For this review, take the finished solid that the model builds, in its own axes (mm). Face numbers are marked on the shaded views. Round coordinates to 2 decimals unless told otherwise and drop trailing zeros. Order: outer loops, then holes, each group sorted by start corner. A loop starts at its lowest first (then second) coordinate and runs counter-clockwise, first axis right, second up. Notation, with made-up numbers: M -1.75,-13.75 L 45.25,-13.75 A31 cw 45.25,24.25 Z; hole C 74,-5.5 d3. An arc over 180 degrees is marked long. Use a Markdown table: item, result.
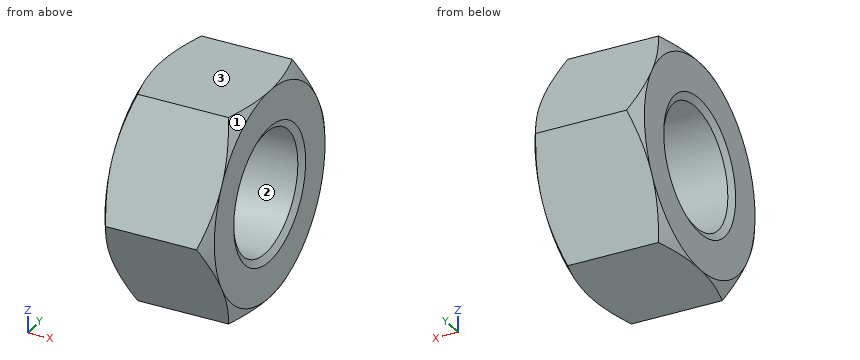
Autodesk Inventor part; units mm, degrees
ref_plane "Work Plane1" through (-87.2182, 0, 0) normal (0, -0.8660254, -0.5) x (1, 0, 0)
ref_plane "YZ Plane" through (0, 0, 0) normal (1, 0, 0) x (0, 1, 0)
ref_plane "XZ Plane" through (0, 0, 0) normal (0, 1, 0) x (-1, 0, 0)
sketch "Sketch1" plane through (0, 0, 0) normal (1, 0, 0) x (0, 1, 0)
  line L0 (-46.188, 0) -> (-23.094, 40)
  line L1 (-23.094, 40) -> (23.094, 40)
  line L2 (23.094, 40) -> (46.188, 0)
  line L3 (46.188, 0) -> (23.094, -40)
  line L4 (23.094, -40) -> (-23.094, -40)
  line L5 (-23.094, -40) -> (-46.188, 0)
  point P0 (0, 0)
  point P1 (0, 0)
  dimension "d0" = 92.376
extrude "Body" add sketch "Sketch1" along normal blind 42
sketch "Sketch2" plane through (0, 0, 0) normal (0, 0, 1) x (1, 0, 0)
  line L0 (0, 23.094) -> (0, 46.188)
  line L1 (0, 46.188) -> (42, 46.188)
  line L2 (42, 23.094) -> (42, 46.188)
  line L3 (-8.4, 0) -> (50.4, 0)
  line L4 (3.5727, 46.188) -> (0, 40)
  line L5 (38.4273, 46.188) -> (42, 40)
  dimension "d3" = 30
  dimension "d4" = 30
  dimension "d5" = 80
  dimension "d6" = 80
revolve "Chamfer1" cut sketch "Sketch2" angle 360 about axis through (-10, 0, 0) along (1, 0, 0)
sketch "Sketch3" plane through (42, 0, 0) normal (1, 0, 0) x (0, 0, -1)
  arc A0 (-20, -34.641) -> (20, -34.641) centre (0, 0) ccw
hole "Thread" at (42, 0, 0) direction (-1, 0, 0) diameter 46.5873 end through all
chamfer "Chamfer2" distance 2.7063 angle 30 1 edges at (42, 0, 23.2937) measured on face at (42, -34.2285, -0.9359)
chamfer "Chamfer3" distance 2.7063 angle 30 1 edges at (0, 0, 23.2937) measured on face at (0, -34.2285, -0.9359)
ref_plane "Work Plane1" through (-87.2182, 0, 0) normal (0, -0.8660254, -0.5) x (1, 0, 0)
equation "\"d0\" = 1.1547 * SW"
equation "\"d1\" = KOH"
equation "\"d8\" = -0.5 * GD1 + 0.5 * NND"
equation "\"d40\" = -0.5 * GD1 + 0.5 * NND"
equation "\"d10\" = -0.5 * GD1 + 0.5 * NND"
equation "\"d41\" = -0.5 * GD1 + 0.5 * NND"
equation "\"d3\" = ANG1"
equation "\"d4\" = ANG2"
equation "\"d5\" = SW0"
equation "\"d6\" = SW01"
equation "\"ANG1\" = 30deg"
equation "\"ANG2\" = ANG1"
equation "\"NND\" = 52"
equation "\"KOH\" = 42"
equation "\"SW0\" = SW"
equation "\"SW01\" = SW"
equation "\"GUL\" = 0.541266 * PTC"
equation "\"THREADDIA\" = 52"
equation "\"TOA\" = 30deg"
equation "\"PTC\" = 5"
equation "\"E0\" = 1.155 * SW"
equation "\"GAL\" = 0.541266 * PTC"
properties part number "BS 3692 - M52" material "Steel, Mild"
Q1. Draft analysis for pull direction Y (two halves, no side actions). For the marked faces 1, 2 and 3, state which applies: pulls with the +Y half, pulls with the -Y half, needs draft (parallel to the pull), parting line crosses it, or undercut.
Determined:
| item | result |
|---|---|
| face 1 | pulls with the -Y half |
| face 2 | undercut |
| face 3 | needs draft |
Q2. Clearance check with flat-ended pins moving along their axes: pin 1 (1.5 mm diameter, centred on x = 7, y = 29, fed in from -Z); pin 2 (4 mm diameter, centred on x = 16, z = -31, fed in from +Y); pin 3 (5 mm diameter, centred on y = -30.5, z = -31, fed in from +X); pin 4 (10 mm diameter, centred on x = 19, y = -27, fed in from +Z). State where each tip first meets the part, or that it passes through.
Determined:
| item | result |
|---|---|
| pin 1 | stops at z = -31.07 |
| pin 2 | stops at y = 29.44 |
| pin 3 | stops at x = 41.43 |
| pin 4 | stops at z = 40 |
Q3. Wall thickness on line 1 along Z through (x, y) = (14.5, 0); line 2 along Y through (x, z) = (30.5, 0); line 3 along Z through (x, y) = (16, -3): over which ranges is each line inside the solid? List them lowest first. Write a range as [from, to].
Determined:
| item | result |
|---|---|
| line 1 | z = [-40, -23.29], [23.29, 40] |
| line 2 | y = [-46.19, -23.29], [23.29, 46.19] |
| line 3 | z = [-40, -23.1], [23.1, 40] |
Q4. Add section A-A (x = 33). Write out the cut boundary in (y, z), then the cut area to 3 significant figures.
Determined:
| item | result |
|---|---|
| outline | M -46.19,0 L -23.09,-40 L 23.09,-40 L 46.19,0 L 23.09,40 L -23.09,40 Z; hole C 0,0 d46.59 |
| area | 3,840 mm^2 |
